```python
from build123d import *

# Parameters (mm, degrees)
SKETCH_1_W             = 95
SKETCH_1_H             = 65
EXTRUDE_220_DEPTH      = 15
SKETCH_2_W             = 93
SKETCH_2_H             = 63
CUT_EXTRUDE_347_DEPTH  = 14
SKETCH_3_W             = 17
SKETCH_3_H             = 1
ETHERNET_DEPTH         = 13
FILLET_1_R             = 1
FILLET_2_R             = 1
FILLET_3_R             = 1
FILLET_4_R             = 1
SKETCH_4_W             = 8
SKETCH_4_H             = 1
USB_DEPTH              = 4
SKETCH_5_W             = 12
SKETCH_5_H             = 1
MICROSD_DEPTH          = 3
SKETCH_7_W             = 55
SKETCH_7_H             = 37
EXTRUDE_1830_DEPTH     = 10
SKETCH_6_W             = 53
SKETCH_6_H             = 35
CUT_EXTRUDE_1960_DEPTH = 9
SKETCH_8_W             = 35
SKETCH_8_H             = 37
CUT_EXTRUDE_8_DEPTH    = 1


with BuildPart() as part:
    # Эскиз1 → Extrude 220 (new body)
    with BuildSketch(Plane.XY):
        with Locations((47.5, 32.5)):
            Rectangle(SKETCH_1_W, SKETCH_1_H)
    extrude(amount=EXTRUDE_220_DEPTH)

    # Эскиз2 → Cut-Extrude 347 (cut)
    with BuildSketch(Plane.XY.offset(15)):
        with Locations((47.5, 32.5)):
            Rectangle(SKETCH_2_W, SKETCH_2_H)
    extrude(amount=-CUT_EXTRUDE_347_DEPTH, mode=Mode.SUBTRACT)

    # Эскиз3 → Ethernet (cut)
    with BuildSketch(Plane.XY.offset(15)):
        with Locations((80.5, 64.5)):
            Rectangle(SKETCH_3_W, SKETCH_3_H)
    extrude(amount=-ETHERNET_DEPTH, mode=Mode.SUBTRACT)

    # Скругление1
    fillet_1_edges = [part.edges().sort_by_distance(p)[0] for p in [
        (47.5, 65, 0),
    ]]
    fillet(fillet_1_edges, radius=FILLET_1_R)

    # Скругление2
    fillet_2_edges = [part.edges().sort_by_distance(p)[0] for p in [
        (0, 32, 0),
        (0, 64.707106781, 0.292893219),
        (0, 65, 8),
    ]]
    fillet(fillet_2_edges, radius=FILLET_2_R)

    # Скругление3
    fillet_3_edges = [part.edges().sort_by_distance(p)[0] for p in [
        (48, 0, 0),
        (0.292893219, 0, 0.292893219),
        (0, 0, 8),
    ]]
    fillet(fillet_3_edges, radius=FILLET_3_R)

    # Скругление4
    fillet_4_edges = [part.edges().sort_by_distance(p)[0] for p in [
        (95, 64.707106781, 0.292893219),
        (95, 32.5, 0),
        (95, 0.292893219, 0.292893219),
        (95, 65, 8),
        (95, 0, 8),
    ]]
    fillet(fillet_4_edges, radius=FILLET_4_R)

    # Эскиз4 → USB (cut)
    with BuildSketch(Plane.XY.offset(15)):
        with Locations((10.5, 64.5)):
            Rectangle(SKETCH_4_W, SKETCH_4_H)
    extrude(amount=-USB_DEPTH, mode=Mode.SUBTRACT)

    # Эскиз5 → MicroSD (cut)
    with BuildSketch(Plane.XY.offset(15)):
        with Locations((41, 64.5)):
            Rectangle(SKETCH_5_W, SKETCH_5_H)
    extrude(amount=-MICROSD_DEPTH, mode=Mode.SUBTRACT)

    # Эскиз7 → Extrude 1830 (add)
    with BuildSketch(Plane(origin=(0, 0, 0), x_dir=(-1, 0, 0), z_dir=(0, 0, -1))):
        with Locations((-33.5, 24.5)):
            Rectangle(SKETCH_7_W, SKETCH_7_H)
    extrude(amount=-EXTRUDE_1830_DEPTH)

    # Эскиз6 → Cut-Extrude 1960 (cut)
    with BuildSketch(Plane(origin=(0, 0, 0), x_dir=(-1, 0, 0), z_dir=(0, 0, -1))):
        with Locations((-33.5, 24.5)):
            Rectangle(SKETCH_6_W, SKETCH_6_H)
    extrude(amount=-CUT_EXTRUDE_1960_DEPTH, mode=Mode.SUBTRACT)

    # Эскиз8 → Вытянуть8 (cut)
    with BuildSketch(Plane.XY.offset(10)):
        with Locations((43.5, 24.5)):
            Rectangle(SKETCH_8_W, SKETCH_8_H)
    extrude(amount=-CUT_EXTRUDE_8_DEPTH, mode=Mode.SUBTRACT)


solid = part.part
```
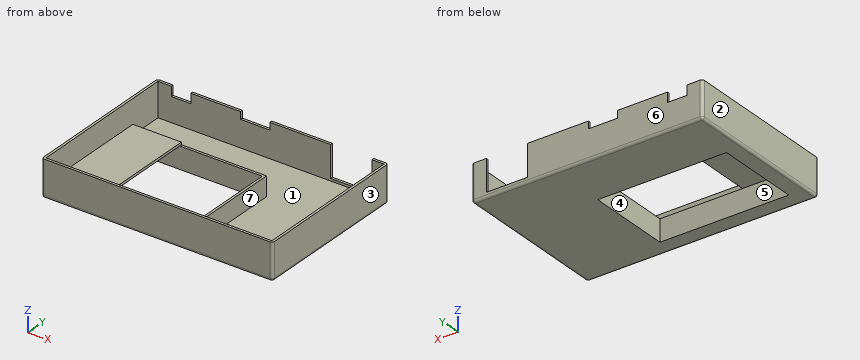
Build history of the part. All positions in model axes, mm. Face numbers are marked on the shaded views. A direction names the side the tool comes from. Coordinates: 2 decimals unless noted, no trailing zeros. Order: outer loops, then holes, each group sorted by start corner. A loop starts at its lowest first (then second) coordinate and runs counter-clockwise, first axis right, second up.
Item 1: Drop flat-ended pins along their axis: pin 1 Ø0.5 at (y, z) = (64.5, 10) entering from -X; pin 2 Ø10 at (x, y) = (19, 20) entering from +Z; pin 3 Ø1.1 at (x, y) = (11.5, 64.5) entering from +Z. Give the stop position or say it passes through.
Filled in:
pin 1: stops at x = 0.03
pin 2: stops at z = 10
pin 3: stops at z = 11
Item 2: Drill centre lines: L1, parallel to X at y = 9, z = 5.5; L2, parallel to Y at x = 53, z = 7.5; L3, parallel to X at y = 6.5, z = 2.75. Where is each one in solid material? Low to high.
Filled in:
L1: x = 0 to 1, 6 to 7, 60 to 61, 94 to 95
L2: y = 0 to 1, 6 to 7, 42 to 43, 64 to 65
L3: x = 0 to 1, 6 to 61, 94 to 95
Item 3: Saw through at B-B on z = 4. List the corners of the cut face in (x, y), then the cut area to 3 significant figures.
Filled in:
outline: (0, 1) arc R1 ccw to (1, 0) - (94, 0) arc R1 ccw to (95, 1) - (95, 64) arc R1 ccw to (94, 65) - (89, 65) - (89, 64) - (94, 64) - (94, 1) - (1, 1) - (1, 64) - (72, 64) - (72, 65) - (1, 65) arc R1 ccw to (0, 64) - close; (6, 6) - (61, 6) - (61, 43) - (6, 43) - close; hole (7, 7) - (60, 7) - (60, 42) - (7, 42) - close
area: 478 mm2
Item 4: Mould opens along X. For the marked faces 1, 2 and 3 say: released by +X, released by -X, zero draft, split by the parting line, or undercut.
Filled in:
face 1: undercut
face 2: released by -X
face 3: released by +X
Item 5: Saw through at D-D on x = 83.5. List the corners of the cut face in (y, z).
Filled in:
outline: (0, 1) arc R1 ccw to (1, 0) - (64, 0) arc R1 ccw to (65, 1) - (65, 2) - (64, 2) - (64, 1) - (1, 1) - (1, 15) - (0, 15) - close
Item 6: Tool access for the marked faces 4, 5, 6 and 7: list every direction of +Z, -Z, +X, -X, +Y, -Y with a clear straight run to the whole face (end or side of a thin tool).
Filled in:
face 4: +Z, -Z
face 5: -Z
face 6: +Z, -Z, +X, -X, +Y
face 7: +Z
Item 7: Saw through at A-A on x = 39.5. List the corners of the cut face in (y, z), then the cut area to 3 significant figures.
Filled in:
outline: (0, 1) arc R1 ccw to (1, 0) - (7, 0) - (7, 9) - (6, 9) - (6, 1) - (1, 1) - (1, 15) - (0, 15) - close; (42, 0) - (64, 0) arc R1 ccw to (65, 1) - (65, 12) - (64, 12) - (64, 1) - (43, 1) - (43, 9) - (42, 9) - close
area: 70.6 mm2
Item 8: Saw through at C-C on y = 9.5. List the corners of the cut face in (x, z).
Filled in:
outline: (0, 1) arc R1 ccw to (1, 0) - (7, 0) - (7, 9) - (26, 9) - (26, 10) - (6, 10) - (6, 1) - (1, 1) - (1, 15) - (0, 15) - close; (60, 0) - (94, 0) arc R1 ccw to (95, 1) - (95, 15) - (94, 15) - (94, 1) - (61, 1) - (61, 9) - (60, 9) - close
